```python
from build123d import *


with BuildPart() as part:
    # Sketch1 → Revolve1 (revolve)
    with BuildSketch(Plane.XY, mode=Mode.PRIVATE) as revolve1_sk:
        with BuildLine():
            Line((2.1, 4), (2.1, 3.8))
            Line((2.1, 3.8), (3, 3.8))
            Line((3, 3.8), (3, 4))
            Line((3, 4), (9.7, 4))
            ThreePointArc((9.7, 4), (9.912132034, 4.087867966), (10, 4.3))
            Line((10, 4.3), (10, 5.5))
            Line((10, 5.5), (10.5, 6))
            Line((10.5, 6), (107.5, 6))
            Line((107.5, 6), (108, 5.5))
            Line((108, 5.5), (108, 5.3))
            ThreePointArc((108, 5.3), (108.087867966, 5.087867966), (108.3, 5))
            Line((108.3, 5), (143.5, 5))
            Line((143.5, 5), (144, 4.5))
            Line((144, 4.5), (144, 4.2))
            ThreePointArc((144, 4.2), (144.058578644, 4.058578644), (144.2, 4))
            Line((144.2, 4), (158.5, 4))
            Line((158.5, 4), (159, 3.5))
            Line((159, 3.5), (159, 0))
            Line((159, 0), (0, 0))
            Line((0, 0), (0, 3.5))
            Line((0, 3.5), (0.5, 4))
            Line((0.5, 4), (2.1, 4))
        make_face()
    revolve(revolve1_sk.sketch.rotate(Axis((-7.5, 0, 0), (1, 0, 0)), 90), axis=Axis((-7.5, 0, 0), (1, 0, 0)))


solid = part.part
```
Design review of the part built by this model. Coordinates are the model's own, in mm. A direction names the side the tool comes from. Coordinates: 2 decimals unless noted, no trailing zeros. Order: outer loops, then holes, each group sorted by start corner. A loop starts at its lowest first (then second) coordinate and runs counter-clockwise, first axis right, second up.
1) Clearance check with flat-ended pins moving along their axes: pin 1 (1 mm diameter, centred on x = 106, z = 3, fed in from +Y); pin 2 (6 mm diameter, centred on x = 94.5, y = 4, fed in from -Z); pin 3 (1 mm diameter, centred on y = -3.5, z = -3.5, fed in from -X). State where each tip first meets the part, or that it passes through.
2) Wall thickness on line 1 along X through (y, z) = (-5, -1.5); line 2 along Y through (x, z) = (127, -3.25); line 3 along Y through (x, z) = (23.5, 0.5): over which ranges is each line inside the solid? List them lowest first.
3) Mouldability with a two-part tool opening along X and no side actions: class faces 1 (the flat face through (10, 4, -2)), 2 (the cylindrical face through (151.45, 3.905, -0.867)), 3 (the cylindrical face through (2.556, -1.141, 3.625)) as +X half, -X half, draft (parallel to the pull), parting line (faces both ways), or undercut.
4) Take a section at B-B, the plane x = 94.5. Give the boundary of the cut face in (y, z).
5) For faces 4 (the flat face through (0, 0, 0)), 5 (the cylindrical face through (6.397, 3.905, -0.867)), 6 (the cylindrical face through (126, 0, -5)), list the 3-axis set-ups (+Z, -Z, +X, -X, +Y, -Y) from which the entire face can be reached by the end or side of a thin tool; tool diameter is ignored.
6) Take a section at A-A, the plane x = 122.5. Give the boundary of the cut face in (y, z).
Returned:
1. pin 1: stops at y = 5.45
1. pin 2: stops at z = -5.92
1. pin 3: stops at x = 10
2. line 1: x = 10 to 108.01
2. line 2: y = -3.8 to 3.8
2. line 3: y = -5.98 to 5.98
3. face 1: -X half
3. face 2: draft
3. face 3: undercut
4. outline: circle Ø12 at (0, 0)
5. face 4: +Z, -Z, -X, +Y, -Y
5. face 5: -X
5. face 6: +X
6. outline: circle Ø10 at (0, 0)
